Geometry check sheet. Reference: the model listing, model coordinates, mm. A direction names the side the tool comes from. Round coordinates to 2 decimals unless told otherwise and drop trailing zeros. Order: outer loops, then holes, each group sorted by start corner. A loop starts at its lowest first (then second) coordinate and runs counter-clockwise, first axis right, second up. Notation, with made-up numbers: (57, 39.5) -> (81, 39.5) arc R13 ccw to (81, 57.5) -> close; hole circle Ø5 at (64, 69.25). An arc over 180 degrees is marked (long way). Use a Markdown table: item, result. Add a question column.
Item 1: Sectioned sample at A-A, the plane z = -141. Record the cut outline in (x, y).
Item 2: Sectioned sample at B-B, the plane x = 12.7. State how many separate pieces and enclosed holes the cut face has, and give its area (3 significant figures).
Item 3: Gauge pin test, flat ends, axial feed: pin 1 Ø12.5 at (x, y) = (8, 87) entering from +Z; pin 2 Ø4.5 at (x, z) = (18, -206) entering from -Y; pin 3 Ø5 at (x, y) = (14.5, 184) entering from -Z; pin 4 Ø10 at (x, z) = (19, -64) entering from -Y. Record the tip position at first contact, or that the pin passes through.
Item 4: Mould release check, pull along Y, two halves, no side actions. Record for faces 4 (the flat face through (19, 286, -195.754)), 5 (the flat face through (13, -282.601, -203)), 6 (the flat face through (16, 80, -68.754)): pulls with the +Y half, pulls with the -Y half, needs draft (parallel to the pull), parting line crosses it, or undercut.
Item 5: Material ranges on probe 1 along Y at (x, z) = (12.7, -97); probe 2 along Z at (x, y) = (12, 204); probe 3 along Z at (x, y) = (7.25, -195), recorded low to high. Write a range as [from, to].
Item 6: Sectioned sample at C-C, the plane z = -164.5. Record the cut outline in (x, y).
Item 7: Set-up check for faces 1 (the flat face through (16, -301, -195.754)), 2 (the cylindrical face through (11.32, -199.9, -183.07)), 3 (the flat face through (13, -79.401, -203)): record each of +Z, -Z, +X, -X, +Y, -Y from which the full face is reachable in a straight line by a thin tool's end or side.
from build123d import *

# Parameters (mm, degrees)
F0_W      = 609.6
F0_H      = 153.9875
F1_DEPTH  = 25.4
F2_W      = 25.4
F2_H      = 12.7
F2_H_2    = 15.875
F3_DEPTH  = 25.4
F7_R      = 6.35
F6_R      = 6.35
F5_R      = 6.35
F4_R      = 6.35
F8_DEPTH  = 177.8
F9_DEPTH  = 1.5875
F12_R     = 6.35
F11_R     = 6.35
F10_R     = 6.35
F13_DEPTH = 177.8
F14_R     = 25.4
F15_DEPTH = 25.4
F16_DEPTH = 76.2
F17_DEPTH = 25.4


with BuildPart() as f1:
    # F0 (on Right) → F1 (new body)
    with BuildSketch(Plane.YZ):
        with Locations((-3.2007116824, -133.0477804439)):
            Rectangle(F0_W, F0_H)
    extrude(amount=F1_DEPTH)

    # F2 (on face) → F3 (cut)
    with BuildSketch(Plane.YZ.offset(25.4)):
        with Locations((-295.3007116824, -62.4040304439)):
            Rectangle(F2_W, F2_H)
        with Locations((-295.3007116824, -202.1040304439)):
            Rectangle(F2_W, F2_H_2)
        with Locations((-92.1007116824, -202.1040304439)):
            Rectangle(F2_W, F2_H_2)
        with Locations((-92.1007116824, -62.4040304439)):
            Rectangle(F2_W, F2_H)
        with Locations((85.6992883176, -62.4040304439)):
            Rectangle(F2_W, F2_H)
        with Locations((85.6992883176, -202.1040304439)):
            Rectangle(F2_W, F2_H_2)
        with Locations((288.8992883176, -62.4040304439)):
            Rectangle(F2_W, F2_H)
        with Locations((288.8992883176, -202.1040304439)):
            Rectangle(F2_W, F2_H_2)
    extrude(amount=-F3_DEPTH, mode=Mode.SUBTRACT)

    # F7 (on face) + F6 (on face) + F5 (on face) + F4 (on face) → F8 (cut)
    with BuildSketch(Plane.XY.offset(-68.7540304439)):
        with Locations((12.7, 288.8992883176)):
            Circle(F7_R)
    with BuildSketch(Plane.XY.offset(-68.7540304439)):
        with Locations((12.7, 85.6992883176)):
            Circle(F6_R)
    with BuildSketch(Plane.XY.offset(-68.7540304439)):
        with Locations((12.7, -92.1007116824)):
            Circle(F5_R)
    with BuildSketch(Plane.XY.offset(-68.7540304439)):
        with Locations((12.7, -295.3007116824)):
            Circle(F4_R)
    extrude(amount=-F8_DEPTH, mode=Mode.SUBTRACT)

    # F9 (add): faces of the model
    f9_faces = [f1.faces().sort_by_distance(p)[0] for p in [
        (12.7, -282.9599219273, -194.1665304439),
        (12.7, -79.7599219273, -194.1665304439),
        (12.7, 98.0400780727, -194.1665304439),
        (12.7, 301.2400780727, -194.1665304439),
    ]]
    extrude(f9_faces, amount=F9_DEPTH)

    # F12 (on face) + F11 (on face) + F10 (on face) → F13 (cut)
    with BuildSketch(Plane.XY.offset(-56.0540304439)):
        with Locations((12.7, -193.7007116824)):
            Circle(F12_R)
    with BuildSketch(Plane.XY.offset(-56.0540304439)):
        with Locations((12.7, -3.2007116824)):
            Circle(F11_R)
    with BuildSketch(Plane.XY.offset(-56.0540304439)):
        with Locations((12.7, 187.2992883176)):
            Circle(F10_R)
    extrude(amount=-F13_DEPTH, mode=Mode.SUBTRACT)

    # F14 (on face) → F15 (cut)
    with BuildSketch(Plane.YZ.offset(25.4)):
        with Locations((-193.7007116824, -132.2540304439)):
            Circle(F14_R)
        with Locations((187.2992883176, -132.2540304439)):
            Circle(F14_R)
    extrude(amount=-F15_DEPTH, mode=Mode.SUBTRACT)

    # F12 (on face) + F10 (on face) → F16 (join)
    with BuildSketch(Plane.XY.offset(-56.0540304439)):
        with Locations((12.7, -193.7007116824)):
            Circle(F12_R)
    with BuildSketch(Plane.XY.offset(-56.0540304439)):
        with Locations((12.7, 187.2992883176)):
            Circle(F10_R)
    extrude(amount=-F16_DEPTH)

    # F14 (on face) → F17 (cut)
    with BuildSketch(Plane.YZ.offset(25.4)):
        with Locations((-193.7007116824, -132.2540304439)):
            Circle(F14_R)
        with Locations((187.2992883176, -132.2540304439)):
            Circle(F14_R)
    extrude(amount=-F17_DEPTH, mode=Mode.SUBTRACT)


solid = f1.part
Found:
| question | item | result |
|---|---|---|
| 1 | outline | (0, -308) -> (25.4, -308) -> (25.4, -217.55) -> (0, -217.55) -> close; (0, -169.85) -> (25.4, -169.85) -> (25.4, 163.45) -> (0, 163.45) -> close; (0, 211.15) -> (25.4, 211.15) -> (25.4, 301.6) -> (0, 301.6) -> close; hole circle Ø12.7 at (12.7, -295.3); hole circle Ø12.7 at (12.7, -92.1); hole circle Ø12.7 at (12.7, -3.2); hole circle Ø12.7 at (12.7, 85.7); hole circle Ø12.7 at (12.7, 288.9) |
| 2 | separate pieces | 6 |
| 2 | enclosed holes | 0 |
| 2 | area | 77,300 mm2 |
| 3 | pin 1 | stops at z = -68.75 |
| 3 | pin 2 | stops at y = -282.6 |
| 3 | pin 3 | stops at z = -107.52 |
| 3 | pin 4 | stops at y = -308 |
| 4 | face 4 | needs draft |
| 4 | face 5 | pulls with the -Y half |
| 4 | face 6 | undercut |
| 5 | probe 1 | y = [-308, -301.65], [-288.95, -98.45], [-85.75, -9.55], [3.15, 79.35], [92.05, 282.55], [295.25, 301.6] |
| 5 | probe 2 | z = [-210.04, -151.39], [-113.12, -56.05] |
| 5 | probe 3 | z = [-106.89, -56.05] |
| 6 | outline | (0, -308) -> (25.4, -308) -> (25.4, 301.6) -> (0, 301.6) -> close; hole circle Ø12.7 at (12.7, -295.3); hole circle Ø12.7 at (12.7, -193.7); hole circle Ø12.7 at (12.7, -92.1); hole circle Ø12.7 at (12.7, -3.2); hole circle Ø12.7 at (12.7, 85.7); hole circle Ø12.7 at (12.7, 187.3); hole circle Ø12.7 at (12.7, 288.9) |
| 7 | face 1 | -Z, +X, -X, -Y |
| 7 | face 2 | -Z |
| 7 | face 3 | -Z, +X, -X |
